```python
from build123d import *

# Parameters (mm, degrees)
SKETCH1_R           = 3.4
BOSS_EXTRUDE1_DEPTH = 4.6
BOSS_EXTRUDE2_START = -1.9
BOSS_EXTRUDE2_DEPTH = 1.9
SKETCH4_R           = 2.325
CUT_EXTRUDE1_DEPTH  = 2.9
FILLET1_R           = 1
CUT_EXTRUDE2_REACH  = 18.71
SKETCH5_R           = 1.25
SKETCH6_R           = 2.375
CUT_EXTRUDE3_DEPTH  = 0.9
CUT_EXTRUDE4_REACH  = 18.71
SKETCH7_R           = 1


with BuildPart() as part:
    # Sketch1 → Boss-Extrude1 (new body)
    with BuildSketch(Plane(origin=(0, 0, 0), x_dir=(1, 0, 0), z_dir=(0, 1, 0))):
        with Locations(Location((0, 0, 0), (0, 0, 270))):
            Circle(SKETCH1_R)
    extrude(amount=BOSS_EXTRUDE1_DEPTH)

    # Sketch3 → Boss-Extrude2 (add)
    with BuildSketch(Plane(origin=(0, 4.6, 0), x_dir=(1, 0, 0), z_dir=(0, 1, 0)).offset(BOSS_EXTRUDE2_START)):
        with BuildLine():
            Line((-13.973038518, -1.855236037), (-2.053265692, -2.71))
            ThreePointArc((-2.053265692, -2.71), (3.4, 0), (-2.053265692, 2.71))
            Line((-2.053265692, 2.71), (-13.973038518, 1.855236037))
            ThreePointArc((-13.973038518, 1.855236037), (-15.7, 0), (-13.973038518, -1.855236037))
        make_face()
    extrude(amount=BOSS_EXTRUDE2_DEPTH)

    # Sketch4 → Cut-Extrude1 (cut)
    with BuildSketch(Plane.XZ):
        with Locations(Location((0, 0, 0), (0, 0, 270))):
            Circle(SKETCH4_R)
    extrude(amount=-CUT_EXTRUDE1_DEPTH, mode=Mode.SUBTRACT)

    # Fillet1
    fillet1_edges = [part.edges().sort_by_distance(p)[0] for p in [
        (-2.053265692, 3.65, -2.71),
        (-2.053265692, 3.65, 2.71),
    ]]
    fillet(fillet1_edges, radius=FILLET1_R)

    # Sketch5 → Cut-Extrude2 (cut, up to next)
    with BuildSketch(Plane(origin=(0, 4.6, 0), x_dir=(1, 0, 0), z_dir=(0, 1, 0)), mode=Mode.PRIVATE) as cut_extrude2_sk1:
        with Locations(Location((0, 0, 0), (0, 0, 270))):
            Circle(SKETCH5_R)
    cut_extrude2_tool1 = extrude(cut_extrude2_sk1.sketch, amount=-CUT_EXTRUDE2_REACH, mode=Mode.PRIVATE) & part.part
    add(cut_extrude2_tool1.solids().sort_by_distance((0, 4.6, 0))[0], mode=Mode.SUBTRACT)

    # Sketch6 → Cut-Extrude3 (cut)
    with BuildSketch(Plane(origin=(0, 4.6, 0), x_dir=(1, 0, 0), z_dir=(0, 1, 0))):
        with Locations(Location((0, 0, 0), (0, 0, 270))):
            Circle(SKETCH6_R)
    extrude(amount=-CUT_EXTRUDE3_DEPTH, mode=Mode.SUBTRACT)

    # Sketch7 → Cut-Extrude4 (cut, up to next)
    with BuildSketch(Plane(origin=(0, 4.6, 0), x_dir=(1, 0, 0), z_dir=(0, 1, 0)), mode=Mode.PRIVATE) as cut_extrude4_sk1:
        with Locations(Location((-10.7, 0, 0), (0, 0, 270))):
            Circle(SKETCH7_R)
    cut_extrude4_tool1 = extrude(cut_extrude4_sk1.sketch, amount=-CUT_EXTRUDE4_REACH, mode=Mode.PRIVATE) & part.part
    add(cut_extrude4_tool1.solids().sort_by_distance((-10.7, 4.6, 0))[0], mode=Mode.SUBTRACT)


solid = part.part
```
CAD build for the part. Positions are in the model's coordinates, mm. A direction names the side the tool comes from. Round coordinates to 2 decimals unless told otherwise and drop trailing zeros. Loops run counter-clockwise (first coordinate to the right, second up) from the corner with the lowest first, then second, coordinate; pieces in that order, holes last. Notation, with made-up numbers: M 83,-19.5 L 134,-19.5 A7 cw 134,-9.5 Z; hole C -20,26.5 d5. An arc over 180 degrees is marked long. Use a Markdown table: item, result. Add a question column.
(1) Cut at C-C (y = 2.2). Give the cut face in (x, z) (3 decimals), and give its area (3 significant figures).
(2) Cut at A-A (z = 0). Give the cut face in (x, y) (3 decimals).
(3) Which spindle directions (+Z, -Z, +X, -X, +Y, -Y) get a long thin tool onto all of the face, cutting with end or side? Do faces 4 (the face through (0.698, 1.43, -2.218)), 5 (the face through (-1.45, 4.16, -1.88)), 6 (the face through (-11.676, 3.663, -0.217)). Say none if no direction does.
(4) Flat gauge pins, fed straight in: pin 1 (1 mm diameter, centred on x = -10, y = 3.5, fed in from +Z); pin 2 (3 mm diameter, centred on x = 0, z = 0, fed in from +Y); pin 3 (1.5 mm diameter, centred on x = -9, z = -2.5, fed in from -Y). Where does each tip first touch, or does it go through?
(5) Pull direction X, two halves, no side cores. Call faces 1 (the face through (2.867, 2.268, 1.828)), 2 (the face through (-6, 4.6, 0)), 3 (the face through (-1, 3.7, 1)): +X half, -X half, draft (parallel to the pull), parting line (faces both ways), or undercut.
(6) Cut at D-D (x = -10.7). Give the cut face in (y, z), and give its area (3 significant figures).
(7) Cut at B-B (x = 0). Give the cut face in (y, z) (3 decimals).
(8) Drill centre lines: line 1 (X direction, y = 1.05, z = 0) (3 decimals); line 2 (Z direction, x = -1.25, y = 2.7); line 3 (Z direction, x = -0.25, y = 3.2). Where is each one in solid material? Low to high.
Geometry says:
| question | item | result |
|---|---|---|
| 1 | outline | C 0,0 d6.8; hole C 0,0 d4.65 |
| 1 | area | 19.3 mm² |
| 2 | outline | M -15.7,2.7 L -11.7,2.7 L -11.7,4.6 L -15.7,4.6 Z; M -9.7,2.7 L -3.4,2.7 L -3.4,0 L -2.325,0 L -2.325,2.9 L -1.25,2.9 L -1.25,3.7 L -2.375,3.7 L -2.375,4.6 L -9.7,4.6 Z; M 1.25,2.9 L 2.325,2.9 L 2.325,0 L 3.4,0 L 3.4,4.6 L 2.375,4.6 L 2.375,3.7 L 1.25,3.7 Z |
| 3 | face 4 | -Y |
| 3 | face 5 | +Y |
| 3 | face 6 | +Y, -Y |
| 4 | pin 1 | stops at z = 2.18 |
| 4 | pin 2 | stops at y = 3.7 |
| 4 | pin 3 | stops at y = 2.7 |
| 5 | face 1 | parting line |
| 5 | face 2 | draft |
| 5 | face 3 | undercut |
| 6 | outline | M 2.7,-2.09 L 4.6,-2.09 L 4.6,-1 L 2.7,-1 Z; M 2.7,1 L 4.6,1 L 4.6,2.09 L 2.7,2.09 Z |
| 6 | area | 4.14 mm² |
| 7 | outline | M 0,-3.4 L 4.6,-3.4 L 4.6,-2.375 L 3.7,-2.375 L 3.7,-1.25 L 2.9,-1.25 L 2.9,-2.325 L 0,-2.325 Z; M 0,2.325 L 2.9,2.325 L 2.9,1.25 L 3.7,1.25 L 3.7,2.375 L 4.6,2.375 L 4.6,3.4 L 0,3.4 Z |
| 8 | line 1 | x = -3.4 to -2.325, 2.325 to 3.4 |
| 8 | line 2 | z = -3.16 to -1.96, 1.96 to 3.16 |
| 8 | line 3 | z = -3.39 to -1.22, 1.22 to 3.39 |
